Answer from the drawing. Dimensions are ordinates in mm from the lowest x, y and z of the part. Give positions to 0.01 mm unless a question says otherwise; leave off trailing zeros. Loops run counter-clockwise (first coordinate to the right, second up) from the corner with the lowest first, then second, coordinate; pieces in that order, holes last.
Item 1: Consider line 1 along Y through (x, z) = (30, 8.75); line 2 along Y through (x, z) = (10, 7.5); line 3 along X through (y, z) = (9.5, 7). Determine where each line is inside the solid, lowest interval first.
Item 2: Section C-C, the plane z = 4.5 is taken. Give the number of separate pieces and of enclosed holes in the cut face, and give its area (3 significant figures).
Item 3: Section A-A, the plane y = 10 is taken. Give the vertices of the cut face in (x, z).
Item 4: Section B-B, the plane x = 30 is taken. Give the vertices of the cut face in (y, z), and give its area (3 significant figures).
Item 5: This flat-tipped pin is pushed along its axis until it touches: pin 1 Ø2.5 at (x, y) = (20, 20) entering from -Z. Where does it stop, or does it pass through?
Item 6: Section D-D, the plane y = 37 is taken. Give the vertices of the cut face in (x, z), and give its area (3 significant figures).
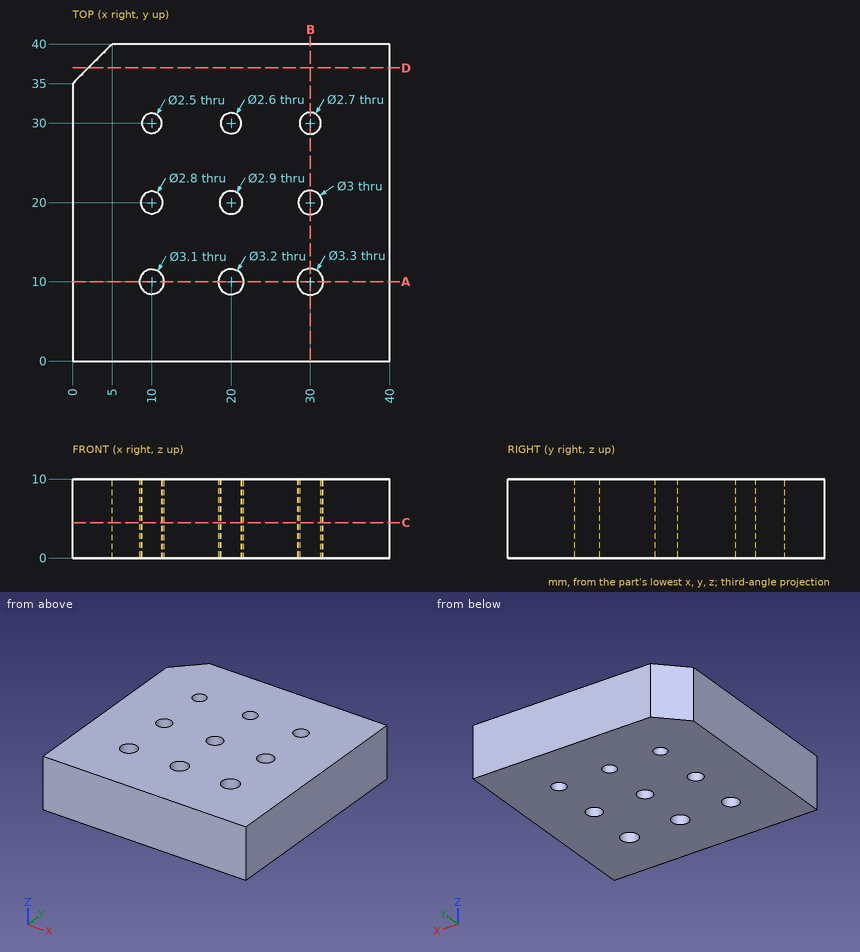
Worked answers:
1. line 1: y = 0 to 8.35, 11.65 to 18.5, 21.5 to 28.65, 31.35 to 40
1. line 2: y = 0 to 8.45, 11.55 to 18.6, 21.4 to 28.75, 31.25 to 40
1. line 3: x = 0 to 8.53, 11.47 to 18.48, 21.52 to 28.43, 31.57 to 40
2. separate pieces: 1
2. enclosed holes: 9
2. area: 1,530 mm2
3. outline: (0, 0) - (8.45, 0) - (8.45, 10) - (0, 10) - close; (11.55, 0) - (18.4, 0) - (18.4, 10) - (11.55, 10) - close; (21.6, 0) - (28.35, 0) - (28.35, 10) - (21.6, 10) - close; (31.65, 0) - (40, 0) - (40, 10) - (31.65, 10) - close
4. outline: (0, 0) - (8.35, 0) - (8.35, 10) - (0, 10) - close; (11.65, 0) - (18.5, 0) - (18.5, 10) - (11.65, 10) - close; (21.5, 0) - (28.65, 0) - (28.65, 10) - (21.5, 10) - close; (31.35, 0) - (40, 0) - (40, 10) - (31.35, 10) - close
4. area: 310 mm2
5. pin 1: passes through
6. outline: (2, 0) - (40, 0) - (40, 10) - (2, 10) - close
6. area: 380 mm2
